Model file for the job. Use its own axes, mm. A direction names the side the tool comes from. Give positions to 0.01 mm unless a question says otherwise; leave off trailing zeros. Loops run counter-clockwise (first coordinate to the right, second up) from the corner with the lowest first, then second, coordinate; pieces in that order, holes last. Notation, with made-up numbers: (25.25, 20) - (58.25, 20) arc R12 cw to (58.25, 31) - close; hole circle Ø10 at (48, 37). An arc over 180 degrees is marked (long way). Use a Markdown table: item, result.
from build123d import *

# Parameters (mm, degrees)
SKETCH1_W                      = 25
SKETCH1_H                      = 53.3
BASE_FLANGE1_DEPTH             = 1.5
EDGE_FLANGE1_STRIP_W           = 9.3
EDGE_FLANGE1_STRIP_H           = 1.5
EDGE_FLANGE1_STRIP_CUT_DEPTH   = 25
EDGE_FLANGE1_STRIP_2_W         = 9.3
EDGE_FLANGE1_STRIP_2_H         = 1.5
EDGE_FLANGE1_STRIP_CUT_2_DEPTH = 25
EDGE_FLANGE1_DEPTH             = 25
EDGE_FLANGE1_BEND_DEPTH        = 25
CUT_EXTRUDE1_REACH             = 78.001
SKETCH12_R                     = 1.5
SKETCH12_R_2                   = 3.25
CUT_EXTRUDE2_REACH             = 78.001
SKETCH13_R                     = 4
SKETCH13_R_2                   = 1.1
FILLET1_R                      = 12.5
SKETCH17_R                     = 1.6
CUT_EXTRUDE3_DEPTH             = 59.30027873
SKETCH18_R                     = 4.75
CUT_EXTRUDE4_DEPTH             = 59.30027873


# Sheet-metal steps are written as plain solids
with BuildPart() as part:
    # Sketch1 → Base-Flange1 (new body)
    with BuildSketch(Plane(origin=(0, 0, 0), x_dir=(1, 0, 0), z_dir=(0, 1, 0))):
        Rectangle(SKETCH1_W, SKETCH1_H)
    extrude(amount=-BASE_FLANGE1_DEPTH)

    # Edge-Flange1 strip (across the edge) → Edge-Flange1 strip cut (cut)
    with BuildSketch(Plane(origin=(12.5, -1.5, 26.65), x_dir=(0, 0, -1), z_dir=(-1, 0, 0))):
        with Locations((-3, -0.75)):
            Rectangle(EDGE_FLANGE1_STRIP_W, EDGE_FLANGE1_STRIP_H)
    extrude(amount=EDGE_FLANGE1_STRIP_CUT_DEPTH, mode=Mode.SUBTRACT)

    # Edge-Flange1 strip 2 (across the edge) → Edge-Flange1 strip cut 2 (cut)
    with BuildSketch(Plane(origin=(-12.5, -1.5, -26.65), x_dir=(0, 0, 1), z_dir=(1, 0, 0))):
        with Locations((-3, -0.75)):
            Rectangle(EDGE_FLANGE1_STRIP_2_W, EDGE_FLANGE1_STRIP_2_H)
    extrude(amount=EDGE_FLANGE1_STRIP_CUT_2_DEPTH, mode=Mode.SUBTRACT)

    # Edge-Flange1 section (across the edge) → Edge-Flange1 (add)
    with BuildSketch(Plane(origin=(12.5, -1.5, 26.65), x_dir=(0, 0, -1), z_dir=(-1, 0, 0))):
        with BuildLine():
            Line((-1.5, 1.65), (-1.5, 48))
            Line((-1.5, 48), (0, 48))
            Line((0, 48), (0, 1.65))
            ThreePointArc((0, 1.65), (0.483273811, 0.483273811), (1.65, 0))
            Line((1.65, 0), (1.65, -1.5))
            ThreePointArc((1.65, -1.5), (-0.577386361, -0.577386361), (-1.5, 1.65))
        make_face()
    extrude(amount=EDGE_FLANGE1_DEPTH)

    # Edge-Flange1 section 2 (across the edge) → Edge-Flange1 bend (add)
    with BuildSketch(Plane(origin=(-12.5, -1.5, -26.65), x_dir=(0, 0, 1), z_dir=(1, 0, 0))):
        with BuildLine():
            Line((-1.5, 1.65), (-1.5, 48))
            Line((-1.5, 48), (0, 48))
            Line((0, 48), (0, 1.65))
            ThreePointArc((0, 1.65), (0.483273811, 0.483273811), (1.65, 0))
            Line((1.65, 0), (1.65, -1.5))
            ThreePointArc((1.65, -1.5), (-0.577386361, -0.577386361), (-1.5, 1.65))
        make_face()
    extrude(amount=EDGE_FLANGE1_BEND_DEPTH)

    # Sketch12 → Cut-Extrude1 (cut, up to next)
    with BuildSketch(Plane.XY.offset(28.15), mode=Mode.PRIVATE) as cut_extrude1_sk1:
        with Locations((-4.949747468, -32.050252532)):
            Circle(SKETCH12_R)
    cut_extrude1_tool1 = extrude(cut_extrude1_sk1.sketch, amount=-CUT_EXTRUDE1_REACH, mode=Mode.PRIVATE) & part.part
    # Sketch12 → Cut-Extrude1 (cut, up to next)
    with BuildSketch(Plane.XY.offset(28.15), mode=Mode.PRIVATE) as cut_extrude1_sk2:
        with Locations((4.949747468, -32.050252532)):
            Circle(SKETCH12_R)
    cut_extrude1_tool2 = extrude(cut_extrude1_sk2.sketch, amount=-CUT_EXTRUDE1_REACH, mode=Mode.PRIVATE) & part.part
    # Sketch12 → Cut-Extrude1 (cut, up to next)
    with BuildSketch(Plane.XY.offset(28.15), mode=Mode.PRIVATE) as cut_extrude1_sk3:
        with Locations((-4.949747468, -41.949747468)):
            Circle(SKETCH12_R)
    cut_extrude1_tool3 = extrude(cut_extrude1_sk3.sketch, amount=-CUT_EXTRUDE1_REACH, mode=Mode.PRIVATE) & part.part
    # Sketch12 → Cut-Extrude1 (cut, up to next)
    with BuildSketch(Plane.XY.offset(28.15), mode=Mode.PRIVATE) as cut_extrude1_sk4:
        with Locations((4.949747468, -41.949747468)):
            Circle(SKETCH12_R)
    cut_extrude1_tool4 = extrude(cut_extrude1_sk4.sketch, amount=-CUT_EXTRUDE1_REACH, mode=Mode.PRIVATE) & part.part
    # Sketch12 → Cut-Extrude1 (cut, up to next)
    with BuildSketch(Plane.XY.offset(28.15), mode=Mode.PRIVATE) as cut_extrude1_sk5:
        with Locations((0, -37)):
            Circle(SKETCH12_R_2)
    cut_extrude1_tool5 = extrude(cut_extrude1_sk5.sketch, amount=-CUT_EXTRUDE1_REACH, mode=Mode.PRIVATE) & part.part
    add(cut_extrude1_tool1.solids().sort_by_distance((-4.949747, -32.050253, 28.15))[0], mode=Mode.SUBTRACT)
    add(cut_extrude1_tool2.solids().sort_by_distance((4.949747, -32.050253, 28.15))[0], mode=Mode.SUBTRACT)
    add(cut_extrude1_tool3.solids().sort_by_distance((-4.949747, -41.949747, 28.15))[0], mode=Mode.SUBTRACT)
    add(cut_extrude1_tool4.solids().sort_by_distance((4.949747, -41.949747, 28.15))[0], mode=Mode.SUBTRACT)
    add(cut_extrude1_tool5.solids().sort_by_distance((0, -37, 28.15))[0], mode=Mode.SUBTRACT)

    # Sketch13 → Cut-Extrude2 (cut, up to next)
    with BuildSketch(Plane(origin=(0, 0, -28.15), x_dir=(-1, 0, 0), z_dir=(0, 0, -1)), mode=Mode.PRIVATE) as cut_extrude2_sk1:
        with Locations(Location((0, -37, 0), (0, 0, 90))):
            Circle(SKETCH13_R)
    cut_extrude2_tool1 = extrude(cut_extrude2_sk1.sketch, amount=-CUT_EXTRUDE2_REACH, mode=Mode.PRIVATE) & part.part
    # Sketch13 → Cut-Extrude2 (cut, up to next)
    with BuildSketch(Plane(origin=(0, 0, -28.15), x_dir=(-1, 0, 0), z_dir=(0, 0, -1)), mode=Mode.PRIVATE) as cut_extrude2_sk2:
        with Locations(Location((0, -44, 0), (0, 0, 90))):
            Circle(SKETCH13_R_2)
    cut_extrude2_tool2 = extrude(cut_extrude2_sk2.sketch, amount=-CUT_EXTRUDE2_REACH, mode=Mode.PRIVATE) & part.part
    # Sketch13 → Cut-Extrude2 (cut, up to next)
    with BuildSketch(Plane(origin=(0, 0, -28.15), x_dir=(-1, 0, 0), z_dir=(0, 0, -1)), mode=Mode.PRIVATE) as cut_extrude2_sk3:
        with Locations(Location((-7, -37, 0), (0, 0, 90))):
            Circle(SKETCH13_R_2)
    cut_extrude2_tool3 = extrude(cut_extrude2_sk3.sketch, amount=-CUT_EXTRUDE2_REACH, mode=Mode.PRIVATE) & part.part
    # Sketch13 → Cut-Extrude2 (cut, up to next)
    with BuildSketch(Plane(origin=(0, 0, -28.15), x_dir=(-1, 0, 0), z_dir=(0, 0, -1)), mode=Mode.PRIVATE) as cut_extrude2_sk4:
        with Locations(Location((0, -30, 0), (0, 0, 90))):
            Circle(SKETCH13_R_2)
    cut_extrude2_tool4 = extrude(cut_extrude2_sk4.sketch, amount=-CUT_EXTRUDE2_REACH, mode=Mode.PRIVATE) & part.part
    # Sketch13 → Cut-Extrude2 (cut, up to next)
    with BuildSketch(Plane(origin=(0, 0, -28.15), x_dir=(-1, 0, 0), z_dir=(0, 0, -1)), mode=Mode.PRIVATE) as cut_extrude2_sk5:
        with Locations(Location((7, -37, 0), (0, 0, 90))):
            Circle(SKETCH13_R_2)
    cut_extrude2_tool5 = extrude(cut_extrude2_sk5.sketch, amount=-CUT_EXTRUDE2_REACH, mode=Mode.PRIVATE) & part.part
    add(cut_extrude2_tool1.solids().sort_by_distance((0, -37, -28.15))[0], mode=Mode.SUBTRACT)
    add(cut_extrude2_tool2.solids().sort_by_distance((0, -44, -28.15))[0], mode=Mode.SUBTRACT)
    add(cut_extrude2_tool3.solids().sort_by_distance((7, -37, -28.15))[0], mode=Mode.SUBTRACT)
    add(cut_extrude2_tool4.solids().sort_by_distance((0, -30, -28.15))[0], mode=Mode.SUBTRACT)
    add(cut_extrude2_tool5.solids().sort_by_distance((-7, -37, -28.15))[0], mode=Mode.SUBTRACT)

    # Fillet1
    fillet1_edges = [part.edges().sort_by_distance(p)[0] for p in [
        (12.5, -49.5, 27.4),
        (-12.5, -49.5, 27.4),
        (-12.5, -49.5, -27.4),
        (12.5, -49.5, -27.4),
    ]]
    fillet(fillet1_edges, radius=FILLET1_R - 0.0001)  # a hair under: the kernel refuses the full size

    # Sketch17 → Cut-Extrude3 (cut, through all)
    with BuildSketch(Plane(origin=(0, 0, 0), x_dir=(1, 0, 0), z_dir=(0, 1, 0))):
        with Locations(Location((-6, 6, 0), (0, 0, 270))):
            Circle(SKETCH17_R)
        with Locations(Location((6, 6, 0), (0, 0, 270))):
            Circle(SKETCH17_R)
        with Locations(Location((6, -6, 0), (0, 0, 270))):
            Circle(SKETCH17_R)
        with Locations(Location((-6, -6, 0), (0, 0, 270))):
            Circle(SKETCH17_R)
    extrude(amount=-CUT_EXTRUDE3_DEPTH, mode=Mode.SUBTRACT)

    # Sketch18 → Cut-Extrude4 (cut, through all)
    with BuildSketch(Plane(origin=(0, 0, 0), x_dir=(1, 0, 0), z_dir=(0, 1, 0))):
        with Locations(Location((0, 0, 0), (0, 0, 270))):
            Circle(SKETCH18_R)
    extrude(amount=-CUT_EXTRUDE4_DEPTH, mode=Mode.SUBTRACT)


solid = part.part
(1) Slice it at A-A, the plane y = -23.5. Write the cut outline in (x, z).
Computed:
| item | result |
|---|---|
| outline | (-12.5, -28.15) - (12.5, -28.15) - (12.5, -26.65) - (-12.5, -26.65) - close; (-12.5, 26.65) - (12.5, 26.65) - (12.5, 28.15) - (-12.5, 28.15) - close |
(2) Drill centre lines: probe 1 along X at (y, z) = (-0.65, 6); probe 2 along X at (y, z) = (-37, -27); probe 3 along Z at (x, y) = (10.75, -5.5). Where is each one in solid material? Low to high. Write a range as [from, to].
Computed:
| item | result |
|---|---|
| probe 1 | [-12.5, -7.6], [-4.4, 4.4], [7.6, 12.5] |
| probe 2 | [-12.5, -8.1], [-5.9, -4], [4, 5.9], [8.1, 12.5] |
| probe 3 | [-28.15, -26.65], [26.65, 28.15] |
(3) Slice it at B-B, the plane z = -6. Write the cut outline in (x, y), plus the area to 3 significant figures.
Computed:
| item | result |
|---|---|
| outline | (-12.5, -1.5) - (-7.6, -1.5) - (-7.6, 0) - (-12.5, 0) - close; (-4.4, -1.5) - (4.4, -1.5) - (4.4, 0) - (-4.4, 0) - close; (7.6, -1.5) - (12.5, -1.5) - (12.5, 0) - (7.6, 0) - close |
| area | 27.9 mm² |
(4) Pin check, flat tips, straight feed: P1, Ø12, axis at x = 2.5, z = 6.5, coming from the +Y side; P2, Ø4, axis at x = 0, y = -37, coming from the -Z side; P3, Ø1.8, axis at x = 7, y = -37, coming from the -Z side; P4, Ø1.8, axis at x = -4.95, y = -32.05, coming from the +Z side. Stop position of each tip, or through.
Computed:
| item | result |
|---|---|
| P1 | y = 0 |
| P2 | through |
| P3 | z = 26.65 |
| P4 | z = -26.65 |
(5) Mould opens along Z. For faces 6 (the cylindrical face through (4.625, -43.414, 27.41)), 7 (the flat face through (0, -26, -28.15)), 8 (the flat face through (0, -27, -26.65)) say: pulls with the +Z half, pulls with the -Z half, needs draft (parallel to the pull), parting line crosses it, or undercut.
Computed:
| item | result |
|---|---|
| face 6 | needs draft |
| face 7 | pulls with the -Z half |
| face 8 | undercut |
(6) Slice it at D-D, the plane x = -9.25. Write the cut outline in (y, z).
Computed:
| item | result |
|---|---|
| outline | (-45.41, -28.15) - (-3.15, -28.15) arc R3.15 ccw to (0, -25) - (0, 25) arc R3.15 ccw to (-3.15, 28.15) - (-45.41, 28.15) - (-45.41, 26.65) - (-3.15, 26.65) arc R1.65 cw to (-1.5, 25) - (-1.5, -25) arc R1.65 cw to (-3.15, -26.65) - (-45.41, -26.65) - close |
(7) 3-axis set-ups, long thin cutter, end or side, ignore diameter. For faces 1 (the cylindrical face through (7.33, -35.95, -27.41)), 2 (the cylindrical face through (4.754, -30.563, 27.41)), 3 (the cylindrical face through (5.39, -0.74, -4.52)), 4 (the cylindrical face through (-0.175, -0.898, -27.203)), 5 (the flat face through (0, -27, 26.65)): which of +Z, -Z, +X, -X, +Y, -Y reach the whole face in a straight line?
Computed:
| item | result |
|---|---|
| face 1 | -Z |
| face 2 | +Z |
| face 3 | +Y, -Y |
| face 4 | -Z, +X, -X, +Y |
| face 5 | +X, -X, -Y |
(8) Slice it at C-C, the plane y = -46. Write the cut outline in (x, z).
Computed:
| item | result |
|---|---|
| outline | (-8.67, -28.15) - (8.67, -28.15) - (8.67, -26.65) - (-8.67, -26.65) - close; (-8.67, 26.65) - (8.67, 26.65) - (8.67, 28.15) - (-8.67, 28.15) - close |
